Geometry check sheet. Reference: the model listing, model coordinates, mm. A direction names the side the tool comes from. Round coordinates to 2 decimals unless told otherwise and drop trailing zeros. Write each loop counter-clockwise with the first axis right and the second up, starting at its lowest first coordinate (ties: lowest second). Pieces come first, ordered by that corner, then holes. Notation, with made-up numbers: (12, 72.5) -> (46, 72.5) arc R10 cw to (46, 90.5) -> close; hole circle Ø10 at (21.5, 59). An arc over 180 degrees is marked (long way). Use a Markdown table: item, result.
```python
from build123d import *

# Parameters (mm, degrees)
SKETCH1_R                   = 15
BOSS_EXTRUDE1_DEPTH         = 2
SKETCH2_R                   = 8
BOSS_EXTRUDE2_DEPTH         = 16
F_3_8_24_TAPPED_HOLE1_D     = 8.4328
F_3_8_24_TAPPED_HOLE1_DEPTH = 24.4
F_3_8_24_TAPPED_HOLE1_TIP   = 2.533468714
SKETCH5_R                   = 1.25
CUT_EXTRUDE1_DEPTH          = 10


with BuildPart() as part:
    # Sketch1 → Boss-Extrude1 (new body)
    with BuildSketch(Plane(origin=(0, 0, 0), x_dir=(1, 0, 0), z_dir=(0, 1, 0))):
        Circle(SKETCH1_R)
    extrude(amount=-BOSS_EXTRUDE1_DEPTH)

    # Sketch2 → Boss-Extrude2 (add)
    with BuildSketch(Plane.XZ.offset(2)):
        Circle(SKETCH2_R)
    extrude(amount=BOSS_EXTRUDE2_DEPTH)

    # 3/8-24 Tapped Hole1
    with Locations(Plane(origin=(0, -18, 0), x_dir=(-1, 0, 0), z_dir=(0, -1, 0))):
        with Locations((0, 0)):
            Hole(F_3_8_24_TAPPED_HOLE1_D / 2, depth=F_3_8_24_TAPPED_HOLE1_DEPTH)
            with Locations((0, 0, -(F_3_8_24_TAPPED_HOLE1_DEPTH + F_3_8_24_TAPPED_HOLE1_TIP / 2))):  # 118° drill point
                Cone(0, F_3_8_24_TAPPED_HOLE1_D / 2, F_3_8_24_TAPPED_HOLE1_TIP, mode=Mode.SUBTRACT)

    # Sketch5 → Cut-Extrude1 (cut)
    with BuildSketch(Plane(origin=(0, 0, 0), x_dir=(1, 0, 0), z_dir=(0, 1, 0))):
        with Locations((11.825, 0)):
            Circle(SKETCH5_R)
        with Locations((-11.825, 0)):
            Circle(SKETCH5_R)
    extrude(amount=-CUT_EXTRUDE1_DEPTH, mode=Mode.SUBTRACT)


solid = part.part
```
(1) Section check A-A on z = 0. Record the cut outline in (x, y) (3 decimals), plus the area to 3 significant figures.
A:
| item | result |
|---|---|
| outline | (-15, -2) -> (-13.075, -2) -> (-13.075, 0) -> (-15, 0) -> close; (-10.575, -2) -> (-8, -2) -> (-8, -18) -> (-4.216, -18) -> (-4.216, 0) -> (-10.575, 0) -> close; (4.216, -18) -> (8, -18) -> (8, -2) -> (10.575, -2) -> (10.575, 0) -> (4.216, 0) -> close; (13.075, -2) -> (15, -2) -> (15, 0) -> (13.075, 0) -> close |
| area | 154 mm2 |
(2) Access from +Z, -Z, +X, -X, +Y, -Y to the whole of each face (thin tool, end or side, straight path). Record for faces 5 (the face through (6, -2, 6)), 6 (the face through (12.98, -0.99, 0.48)).
A:
| item | result |
|---|---|
| face 5 | -Y |
| face 6 | +Y, -Y |
(3) Section check C-C on x = 7.25. Record the cut outline in (y, z), plus the area to 3 significant figures.
A:
| item | result |
|---|---|
| outline | (-18, -3.38) -> (-2, -3.38) -> (-2, -13.13) -> (0, -13.13) -> (0, 13.13) -> (-2, 13.13) -> (-2, 3.38) -> (-18, 3.38) -> close |
| area | 161 mm2 |
(4) Thickness scan on line 1 (Z direction, x = 0, y = -9.5); line 2 (Y direction, x = 12, z = 8.75); line 3 (X direction, y = -10.5, z = -2). Record the ranges inside material, lowest first.
A:
| item | result |
|---|---|
| line 1 | z = -8 to -4.22, 4.22 to 8 |
| line 2 | y = -2 to 0 |
| line 3 | x = -7.75 to -3.71, 3.71 to 7.75 |
(5) Section check B-B on x = 0. Record the cut outline in (y, z), plus the area to 3 significant figures.
A:
| item | result |
|---|---|
| outline | (-18, -8) -> (-2, -8) -> (-2, -15) -> (0, -15) -> (0, -4.22) -> (-18, -4.22) -> close; (-18, 4.22) -> (0, 4.22) -> (0, 15) -> (-2, 15) -> (-2, 8) -> (-18, 8) -> close |
| area | 164 mm2 |
(6) Gauge pin test, flat ends, axial feed: pin 1 Ø8 at (x, z) = (2, -12) entering from +Y; pin 2 Ø8 at (x, y) = (-2.5, -6.5) entering from -Z; pin 3 Ø1.5 at (x, z) = (11.825, 0) entering from +Y; pin 4 Ø2 at (x, y) = (4.5, -9.5) entering from +Z. Record the tip position at first contact, or that the pin passes through.
A:
| item | result |
|---|---|
| pin 1 | stops at y = 0 |
| pin 2 | stops at z = -8 |
| pin 3 | passes through |
| pin 4 | stops at z = 7.19 |
(7) Section check D-D on z = 6.5. Record the cut outline in (x, y), plus the area to 3 significant figures.
A:
| item | result |
|---|---|
| outline | (-13.52, -2) -> (-4.66, -2) -> (-4.66, -18) -> (4.66, -18) -> (4.66, -2) -> (13.52, -2) -> (13.52, 0) -> (-13.52, 0) -> close |
| area | 203 mm2 |
(8) Release check for a two-part mould opening along X. For faces 1 (the face through (-1.73, -9.89, -7.81)), 2 (the face through (-0.55, -8.87, -4.18)), 3 (the face through (-12.75, -0.99, -0.84)), 4 (the face through (3.4, -18, -3.4)) record: +X half, -X half, draft (parallel to the pull), parting line (faces both ways), or undercut.
A:
| item | result |
|---|---|
| face 1 | parting line |
| face 2 | undercut |
| face 3 | undercut |
| face 4 | draft |
